For this review, use the dimensioned drawing (mm, ordinates from the lowest corner) and the shaded views. A direction names the side the tool comes from. Coordinates: 2 decimals unless noted, no trailing zeros. Order: outer loops, then holes, each group sorted by start corner. A loop starts at its lowest first (then second) coordinate and runs counter-clockwise, first axis right, second up. Notation, with made-up numbers: (53, 18.25) -> (103, 18.25) arc R13 ccw to (103, 26.25) -> close; hole circle Ø11 at (-23, -1.5). An arc over 180 degrees is marked (long way). Use CSV: the item, a comma, the result in double quotes. Start each with the question number.
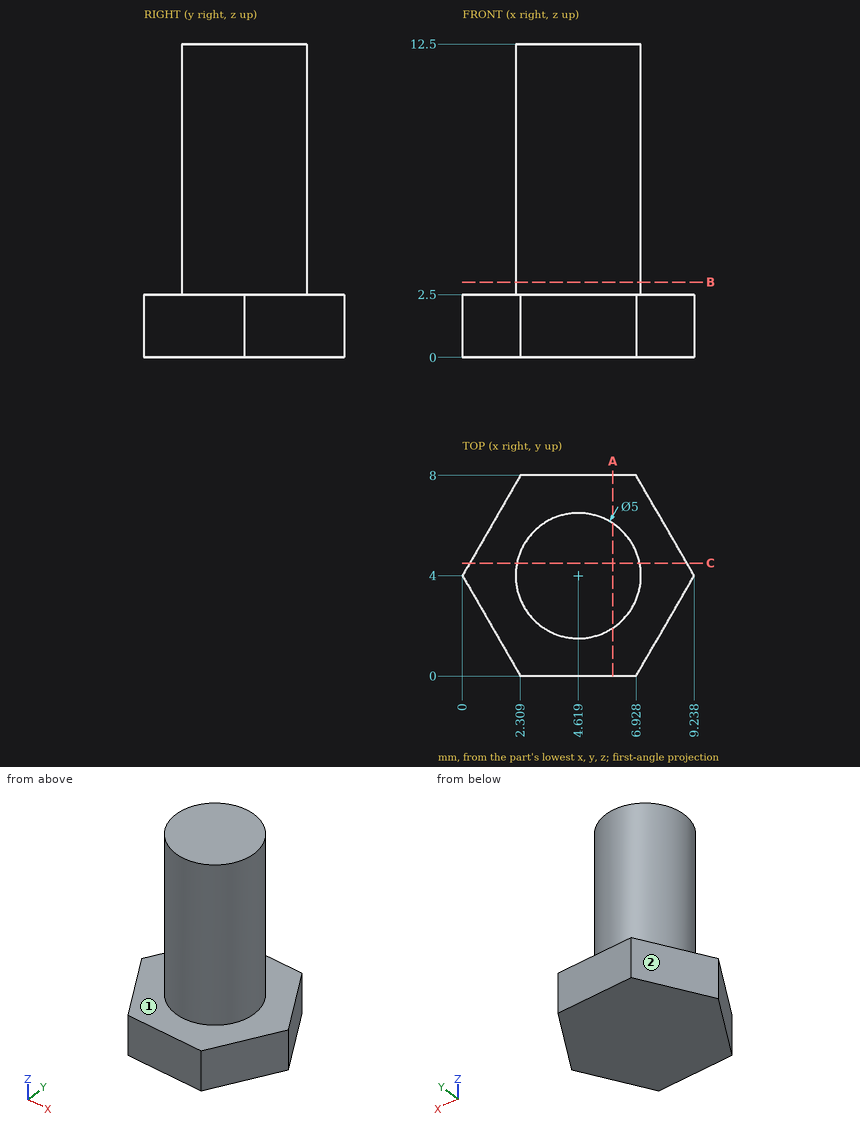
Q1. For the marked faces 1 and 2, list the 3-axis set-ups (+Z, -Z, +X, -X, +Y, -Y) from which the entire face can be reached by the end or side of a thin tool; tool diameter is ignored.
Q2. Add section C-C, the plane y = 4.5. State the section outline as (x, z) points.
Q3. Clearance check with a flat-ended pin moving along its axis: pin 1 Ø3 at (x, z) = (5.5, 7.5) entering from +Y. State where the tip first meets the part, or that it passes through.
Q4. Add section B-B, the plane z = 3. State the section outline as (x, y) points, then the cut area to 3 significant figures.
Q5. To check wall thickness, follow probe 1 along Z at (x, y) = (3.5, 7.5); probe 2 along Y at (x, z) = (4.5, 8.75); probe 3 along Y at (x, z) = (2.75, 11.5). State the ranges of each line that lie inside material, in increasing order.
Q6. Add section A-A, the plane x = 6. State the section outline as (y, z) points.
Answer block:
1,face 1,"+Z"
1,face 2,"+Z, -Z, -X, +Y"
2,outline,"(0.29, 0) -> (8.95, 0) -> (8.95, 2.5) -> (7.07, 2.5) -> (7.07, 12.5) -> (2.17, 12.5) -> (2.17, 2.5) -> (0.29, 2.5) -> close"
3,pin 1,"stops at y = 6.5"
4,outline,"circle Ø5 at (4.62, 4)"
4,area,"19.6 mm²"
5,probe 1,"z = 0 to 2.5"
5,probe 2,"y = 1.5 to 6.5"
5,probe 3,"y = 2.34 to 5.66"
6,outline,"(0, 0) -> (8, 0) -> (8, 2.5) -> (6.08, 2.5) -> (6.08, 12.5) -> (1.92, 12.5) -> (1.92, 2.5) -> (0, 2.5) -> close"
